from build123d import *

# Parameters (mm, degrees)
F1_DEPTH = 5.08


# Not quite as in the source:
# - ends of sketch curves that miss each other by under 0.0002 mm in the source are joined


with BuildPart() as f1:
    # F0 (on Front) → F1 (new body)
    with BuildSketch(Plane.XZ):
        with BuildLine():
            Line((122.3705169674, 43.6478478759), (100.4099901217, 44.7520101639))
            ThreePointArc((100.4099901217, 44.7520101639), (100.0915452408, 44.5649170993), (100.1369538552, 44.1983805872))
            Line((100.1369538552, 44.1983805872), (100.4933528952, 43.3469744222))
            Line((100.4933528952, 43.3469744222), (97.0679359779, 43.3469744222))
            ThreePointArc((97.0679359779, 43.3469744222), (97.1316973251, 43.9112769391), (97.0679359779, 44.4755794561))
            ThreePointArc((97.0679359779, 44.4755794561), (94.352164437, 45.5363400819), (91.4515092493, 45.2416747635))
            ThreePointArc((91.4515092493, 45.2416747635), (83.5169492087, 39.7690696601), (75.469607442, 34.4637006676))
            Line((75.469607442, 34.4637006676), (72.8059848223, 35.5506727573))
            Line((72.8059848223, 35.5506727573), (54.5259908631, 20.9512186051))
            Line((54.5259908631, 20.9512186051), (21.5238705481, 12.7313591723))
            Line((21.5238705481, 12.7313591723), (12.1287463537, 5.188944246))
            Line((12.1287463537, 5.188944246), (-86.8316226794, -10.1466157916))
            Line((-86.8316226794, -10.1466157916), (-122.8382140398, -25.2789985389))
            Line((-122.8382140398, -25.2789985389), (-83.5318863392, -25.8913505822))
            Line((-83.5318863392, -25.8913505822), (13.7389805729, -2.7855467746))
            Line((13.7389805729, -2.7855467746), (24.9590244256, -6.7754736037))
            Line((24.9590244256, -6.7754736037), (59.8014198344, -1.8680947637))
            Line((59.8014198344, -1.8680947637), (74.7804443647, -7.8362995921))
            Line((74.7804443647, -7.8362995921), (77.1637969914, -7.2426764133))
            ThreePointArc((77.1637969914, -7.2426764133), (87.7830978003, -12.7533844887), (99.34301444, -15.8365290594))
            ThreePointArc((99.34301444, -15.8365290594), (102.2935896026, -15.8090472805), (105.1187411592, -14.9574794792))
            ThreePointArc((105.1187411592, -14.9574794792), (105.899310207, -14.1060464291), (106.1757861101, -12.9845357079))
            Line((106.1757861101, -12.9845357079), (106.7682035421, -14.0309760573))
            ThreePointArc((106.7682035421, -14.0309760573), (107.1058211072, -14.2278082292), (107.4434386724, -14.0309760573))
            ThreePointArc((107.4434386724, -14.0309760573), (108.2763784739, -13.0200234045), (108.8199970928, -11.8282630359))
            ThreePointArc((108.8199970928, -11.8282630359), (109.2695277638, -12.0590826755), (109.3121668662, -12.562607687))
            ThreePointArc((109.3121668662, -12.562607687), (109.3974608172, -12.9490474891), (109.7808973473, -13.0469617679))
            ThreePointArc((109.7808973473, -13.0469617679), (111.3986393651, -12.4328774082), (112.8510778468, -11.4923396397))
            ThreePointArc((112.8510778468, -11.4923396397), (113.1573925131, -12.1883188801), (113.9052785257, -12.0509060352))
            Line((113.9052785257, -12.0509060352), (132.3935237104, 0))
            ThreePointArc((132.3935237104, 0), (132.4837449873, 0.8029846441), (132.338838949, 1.5979226652))
            ThreePointArc((132.338838949, 1.5979226652), (133.0482342221, 1.5833492596), (133.4072056247, 2.1953897564))
            Line((133.4072056247, 2.1953897564), (133.4072056247, 5.2268817127))
            ThreePointArc((133.4072056247, 5.2268817127), (133.6969073142, 6.6313363292), (132.2924526977, 6.9210380187))
            Line((132.2924526977, 6.9210380187), (122.3704141488, 3.5393718949))
            ThreePointArc((122.3704141488, 3.5393718949), (121.873706248, 4.0268683816), (121.1812593401, 4.096788644))
            Line((121.1812593401, 4.096788644), (117.4436091822, 3.1937307858))
            ThreePointArc((117.4436091822, 3.1937307858), (117.0266780243, 2.6505498353), (117.0476117867, 1.966123862))
            Line((117.0476117867, 1.966123862), (114.1193957515, 0.3182646199))
            Line((114.1193957515, 0.3182646199), (113.0366831493, 1.4009768977))
            Line((113.0366831493, 1.4009768977), (112.2633179935, 1.4009768977))
            ThreePointArc((112.2633179935, 1.4009768977), (107.0399689979, 13.6404694995), (103.2035150013, 26.3829250952))
            ThreePointArc((103.2035150013, 26.3829250952), (103.4910499167, 30.2221985041), (106.029088113, 33.1172043332))
            ThreePointArc((106.029088113, 33.1172043332), (109.2898552798, 33.4516431179), (112.5333359919, 33.9252301607))
            ThreePointArc((112.5333359919, 33.9252301607), (112.8589818565, 33.5520971563), (112.9913329797, 33.074858591))
            ThreePointArc((112.9913329797, 33.074858591), (113.0214742771, 32.9498651341), (113.1128615921, 32.8594205615))
            ThreePointArc((113.1128615921, 32.8594205615), (114.605495502, 32.7922614875), (116.0903229782, 32.9588558937))
            ThreePointArc((116.0903229782, 32.9588558937), (116.3029445973, 33.0127632591), (116.4383345302, 33.1853422934))
            ThreePointArc((116.4383345302, 33.1853422934), (116.4779468759, 33.679151188), (116.554347608, 34.1686195634))
            Line((116.554347608, 34.1686195634), (119.7698420306, 34.1686195634))
            ThreePointArc((119.7698420306, 34.1686195634), (120.3377346413, 34.0985961328), (120.6763827811, 33.6373773826))
            ThreePointArc((120.6763827811, 33.6373773826), (120.705556032, 33.5058788759), (120.7971017103, 33.4070743991))
            ThreePointArc((120.7971017103, 33.4070743991), (121.8693321552, 33.350668944), (122.933876584, 33.4906863059))
            ThreePointArc((122.933876584, 33.4906863059), (123.0810934781, 33.5938295086), (123.11967467, 33.7693938154))
            ThreePointArc((123.11967467, 33.7693938154), (123.4255269006, 34.1427273195), (123.8907699445, 34.2710721767))
            Line((123.8907699445, 34.2710721767), (125.9903685922, 34.462153965))
            ThreePointArc((125.9903685922, 34.462153965), (126.6924885264, 34.7530229594), (127.1051986302, 35.3911824568))
            Line((127.1051986302, 35.3911824568), (128.2572048943, 38.1039466219))
            ThreePointArc((128.2572048943, 38.1039466219), (128.2729126944, 38.4579608874), (128.0528186952, 38.7356864116))
            Line((128.0528186952, 38.7356864116), (124.5782394715, 41.7643239316))
            Line((124.5782394715, 41.7643239316), (123.9465066021, 41.7643239316))
            Line((123.9465066021, 41.7643239316), (122.3705169674, 43.6478478759))
        make_face()
        with BuildLine():
            Line((70.0165052271, 11.150856785), (76.6579802489, 20.1397516237))
            Line((76.6579802489, 20.1397516237), (80.5816721076, 19.7545750625))
            Line((80.5816721076, 19.7545750625), (91.4935366546, 32.0359588494))
            ThreePointArc((91.4935366546, 32.0359588494), (93.1959095158, 32.0009597447), (94.2558714279, 30.6683761485))
            Line((94.2558714279, 30.6683761485), (91.2971296419, 26.5111941478))
            ThreePointArc((91.2971296419, 26.5111941478), (90.8112616397, 24.8754815968), (91.4297100848, 23.2851530817))
            Line((91.4297100848, 23.2851530817), (93.3299813237, 21.2964983411))
            ThreePointArc((93.3299813237, 21.2964983411), (96.0132194113, 15.5328655264), (97.4206326201, 9.3329931151))
            ThreePointArc((97.4206326201, 9.3329931151), (97.6181949936, 8.6221123526), (98.0063865531, 7.9946654121))
            ThreePointArc((98.0063865531, 7.9946654121), (101.9070751405, 3.1730744617), (104.8498501941, -2.2861549466))
            ThreePointArc((104.8498501941, -2.2861549466), (104.2291914062, -2.8435135125), (104.0495855612, -3.6581346774))
            Line((104.0495855612, -3.6581346774), (105.1997786885, -5.0801357056))
            Line((105.1997786885, -5.0801357056), (100.1594934993, -6.5642189378))
            Line((100.1594934993, -6.5642189378), (82.2009610937, 6.5729623924))
            Line((82.2009610937, 6.5729623924), (78.3157963351, 5.0188977865))
            Line((78.3157963351, 5.0188977865), (70.0165052271, 11.150856785))
        make_face(mode=Mode.SUBTRACT)
    extrude(amount=F1_DEPTH)


solid = f1.part
The model under review builds one solid part; all positions refer to its coordinate system, in mm. A direction names the side the tool comes from. Round coordinates to 2 decimals unless told otherwise and drop trailing zeros. Loops run counter-clockwise (first coordinate to the right, second up) from the corner with the lowest first, then second, coordinate; pieces in that order, holes last. Notation, with made-up numbers: (28, -16.75) -> (82, -16.75) arc R18 cw to (82, -2.75) -> close; hole circle Ø2 at (82.25, 84.5). An arc over 180 degrees is marked (long way). One line per question, with ' | ' between items. Start each with the question number.
Item 1: For pin 1 (4 mm diameter, centred on x = 101, z = -13.5, fed in from +Y); pin 2 (1.7 mm diameter, centred on x = 99, y = -3, fed in from +Z); pin 3 (2.5 mm diameter, centred on x = 119, y = -2, fed in from -Z); pin 4 (2 mm diameter, centred on x = 102, y = -3, fed in from +Z), all flat-tipped, find the tip position at first contact; note any pin that passes through.
Item 2: Wall thickness on line 1 along X through (y, z) = (-1.25, 27.5); line 2 along Z through (x, y) = (70.5, -1.95); line 3 along X through (y, z) = (-4.2, 29): over which ranges is each line inside the solid? List them lowest first. Write a range as [from, to].
Item 3: Machinability: for faces 1 (the face through (19.27, -2.504, -4.753)), 2 (the face through (-36.66, -2.5, -2.37)), 3 (the face through (73.29, -2.5, 15.58)), which of the approach directions +Z, -Z, +X, -X, +Y, -Y give a long, thin tool a straight path to every point of the face, cutting with its end or side? Answer none if there is none.
Item 4: Add section B-B, the plane x = 32.5. Write out the cut boundary in (y, z).
Item 5: Add section A-A, the plane x = -40.5. Write out the cut boundary in (y, z).
Return value:
1) pin 1: stops at y = 0 | pin 2: stops at z = 43.35 | pin 3: stops at z = -9.54 | pin 4: stops at z = 44.72
2) line 1: x = [62.73, 87.46], [92, 103.03] | line 2: z = [-6.13, 10.79], [11.81, 33.71] | line 3: x = [64.6, 88.8], [93.07, 103.12]
3) face 1: -Z, +Y, -Y | face 2: +Z, -X, +Y, -Y | face 3: +Y, -Y
4) outline: (-5.08, -5.71) -> (0, -5.71) -> (0, 15.47) -> (-5.08, 15.47) -> close
5) outline: (-5.08, -15.67) -> (0, -15.67) -> (0, -2.97) -> (-5.08, -2.97) -> close
